Autodesk Inventor part; units mm, degrees
ref_plane "YZ Plane" through (0, 0, 0) normal (1, 0, 0) x (0, 1, 0)
ref_plane "XZ Plane" through (0, 0, 0) normal (0, 1, 0) x (-1, 0, 0)
ref_plane "XY Plane" through (0, 0, 0) normal (0, 0, 1) x (1, 0, 0)
sketch "Náčrt1" plane through (0, 0, 0) normal (0, 0, 1) x (1, 0, 0)
  point P0 (0, 0)
sketch "Náčrt2" plane through (0, 0, 0) normal (0, 0, 1) x (1, 0, 0)
  line L0 (-8.0912, 0) -> (-5.15, 0)
  arc A0 (-0.9091, 8.0399) -> (-8.0912, 0) centre (0, 0) ccw
  line L1 (-0.9091, 8.0399) -> (-0.9091, 5.0691)
  arc A1 (0.9091, 5.0691) -> (-0.9091, 5.0691) centre (0, 0) ccw
  line L2 (0.9091, 5.0691) -> (0.9091, 8.0399)
  arc A2 (8.0912, 0) -> (0.9091, 8.0399) centre (0, 0) ccw
  line L3 (5.15, 0) -> (8.0912, 0)
  arc A3 (4.2917, -2.8468) -> (5.15, 0) centre (0, 0) ccw
  line L4 (4.2917, -2.8468) -> (5.075, -8.7902)
  arc A4 (5.075, -8.7902) -> (-5.075, -8.7902) centre (0, 0) ccw
  line L5 (-4.2917, -2.8468) -> (-5.075, -8.7902)
  arc A5 (-5.15, 0) -> (-4.2917, -2.8468) centre (0, 0) ccw
  line L6 (-16.1, 0) -> (16.1, 0)
  line L7 (0, -14.2512) -> (0, 15.7919)
  dimension "d1" = 0
  dimension "d3" = 5.15
  dimension "d5" = 10.15
  dimension "d7" = 0
  dimension "d9" = 8.0912
  dimension "d11" = 0.9091
  dimension "d13" = 0.9091
  dimension "d15" = 5.075
  dimension "d17" = 5.075
  dimension "d19" = 8.5833
extrude "Vysunutí1" add sketch "Náčrt2" along normal blind 1.1 contours L6 A4 L7 A1 L1 A0 | L0 A5 L5 A4 L6 | A4 L6 A2 L2 A1 L7 | L3 L6 A4 L4 A3
fillet "Zaoblení1" radius 1.3273 4 edges at (-8.0912, 0, 0.55) (-0.9091, 8.0399, 0.55) (0.9091, 8.0399, 0.55) (8.0912, 0, 0.55)
chamfer "Zkosení1" distance 1.015 distance2 1.6222 1 edges at (-5.075, -8.7902, 0.55) measured on face at (-4.4798, 9.1079, 0.7333)
chamfer "Zkosení2" distance 1.6222 distance2 1.015 1 edges at (5.075, -8.7902, 0.55) measured on face at (4.8139, -6.809, 0.3667)
equation "\"d3\" = 0.5 * Diam"
equation "\"d5\" = 0.5 * Diam3"
equation "\"d9\" = 0.294118 * Diam3 + 0.205882 * Diam"
equation "\"d11\" = 0.0909091 * Diam3 - 0.0909091 * Diam"
equation "\"d13\" = 0.0909091 * Diam3 - 0.0909091 * Diam"
equation "\"d15\" = 0.25 * Diam3"
equation "\"d17\" = 0.25 * Diam3"
equation "\"d19\" = 0.833333 * Diam"
equation "\"d20\" = ParT"
equation "\"d22\" = 0.181818 * Diam3 - 0.181818 * sd"
equation "\"d23\" = 0.05 * Diam3"
equation "\"d24\" = 0.222222 * Diam3 - 0.222222 * sd"
equation "\"d25\" = 0.222222 * Diam3 - 0.222222 * sd"
equation "\"d26\" = 0.05 * Diam3"
equation "\"Diam3\" = 20.3"
equation "\"ParT\" = 1.1"
equation "\"Diam\" = 10.3"
equation "\"sd\" = 13"
equation "\"TEMPLATE\" = 1.2345"
properties part number "ANSI B27.7M - 3CMI-13" material "Nerezová ocel"
Could you check a few things on this model? Use its own coordinates, in mm. A direction names the side the tool comes from. Round coordinates to 2 decimals unless told otherwise and drop trailing zeros. Order: outer loops, then holes, each group sorted by start corner. A loop starts at its lowest first (then second) coordinate and runs counter-clockwise, first axis right, second up. Notation, with made-up numbers: M 51,76 L 96,76 A22 cw 96,111 Z; hole C -13.75,63.5 d10. An arc over 180 degrees is marked long. One line per question, with ' | ' between items. Start each with the question number.
(1) Thinking about a two-plate mould opening in Y: for faces 1 (the face through (-7.67, 0.5, 0.56)), 2 (the face through (5.403, -7.718, 0.542)), 3 (the face through (0, 7, 1.1)), which applies, +Y half, -Y half, draft (parallel to the pull), parting line (faces both ways), or undercut?
(2) Suppose I cut it at A-A on x = 7. List the corners of the cut face in (y, z) for me, then the cut area to 3 significant figures.
(3) Suppose I cut it at B-B on y = 3. List the corners of the cut face in (x, z) for me, then the cut area to 3 significant figures.
(4) Suppose I cut it at D-D on y = 5.75. List the corners of the cut face in (x, z) for me.
(5) For faces 4 (the face through (0.909, 5.7, 0.5)), 5 (the face through (0, 7, 0)), 6 (the face through (7.648, 0.473, 0.558)), which set-ups out of +Z, -Z, +X, -X, +Y, -Y let a thin tool reach every point of the face, with its end or its side?
(6) Please list where these lines run through material, in increasing order: line 1 along X through (y, z) = (6.25, 0.55); line 2 along X through (y, z) = (7.5, 0.4); line 3 along X through (y, z) = (-1.25, 0.7).
(7) Suppose I cut it at C-C on z = 0.3. List the corners of the cut face in (x, y) for me, then the cut area to 3 significant figures.
Geometry results:
1) face 1: undercut | face 2: -Y half | face 3: draft
2) outline: M -7.35,0 L 0.05,0 L 0.05,1.1 L -7.35,1.1 Z; M 4.06,0 L 7.35,0 L 7.35,1.1 L 4.06,1.1 Z | area: 11.8 mm²
3) outline: M -9.7,0 L -7.51,0 L -7.51,1.1 L -9.7,1.1 Z; M 7.51,0 L 9.7,0 L 9.7,1.1 L 7.51,1.1 Z | area: 4.80 mm²
4) outline: M -8.36,0 L -5.69,0 L -5.69,1.1 L -8.36,1.1 Z; M -0.91,0 L 0.91,0 L 0.91,1.1 L -0.91,1.1 Z; M 5.69,0 L 8.36,0 L 8.36,1.1 L 5.69,1.1 Z
5) face 4: +Z, -Z, -Y | face 5: -Z, +X, -X, +Y, -Y | face 6: +Z, -Z
6) line 1: -8 to -5.14, -0.91 to 0.91, 5.14 to 8 | line 2: -6.84 to -3.04, -1.52 to 1.52, 3.04 to 6.84 | line 3: -10.07 to -5, 5 to 10.07
7) outline: M -7.93,1.59 A8.09 cw -2.68,7.64 A1.33 cw -0.91,6.38 L -0.91,5.07 A5.15 cw 0.91,5.07 L 0.91,6.38 A1.33 cw 2.68,7.64 A8.09 cw 7.93,1.59 A1.33 cw 6.63,0 L 5.15,0 A5.15 cw 4.29,-2.85 L 4.86,-7.18 L 5.93,-8.24 A10.15 ccw long -5.93,-8.24 L -4.86,-7.18 L -4.29,-2.85 A5.15 cw -5.15,0 L -6.63,0 A1.33 cw Z | area: 134 mm²
